from build123d import *

# Parameters (mm, degrees)
CYLINDER026_R             = 3
CYLINDER026_DEPTH         = 60
CYLINDER026_PITCH_ANGLE   = 90
CYLINDER025_R             = 3
CYLINDER025_DEPTH         = 100
CYLINDER025_ROLL_ANGLE    = 90
CYLINDER027_R             = 3
CYLINDER027_DEPTH         = 60
CYLINDER027_PITCH_ANGLE   = 90
FUSION011_PLACEMENT_ANGLE = 90
BOX026_W                  = 480
BOX026_H                  = 190
BOX026_DEPTH              = 15


with BuildPart() as cylinder032:
    # Cylinder026 → Cylinder026 (new body)
    with BuildSketch(Plane.XY):
        Circle(CYLINDER026_R)
    extrude(amount=CYLINDER026_DEPTH)


with BuildPart() as cylinder032_1:
    # Cylinder026 pitch: moved
    add(cylinder032.part.rotate(Axis((0, 0, 0), (0, 1, 0)), CYLINDER026_PITCH_ANGLE))


with BuildPart() as cylinder032_2:
    # Cylinder026 placement: moved
    add(cylinder032_1.part.moved(Location((-50, -3, 0))))


with BuildPart() as fusion010:
    # Cylinder025 → Cylinder025 (new body)
    with BuildSketch(Plane.XY):
        Circle(CYLINDER025_R)
    extrude(amount=CYLINDER025_DEPTH)


with BuildPart() as fusion010_1:
    # Cylinder025 roll: moved
    add(fusion010.part.rotate(Axis((0, 0, 0), (1, 0, 0)), CYLINDER025_ROLL_ANGLE))


with BuildPart() as fusion010_2:
    # Cylinder025 placement: moved
    add(fusion010_1.part.moved(Location((-50, 0, 0))))

    # Fusion010: union Cylinder032
    add(cylinder032_2.part)


with BuildPart() as handle_top:
    # Cylinder027 → Cylinder027 (new body)
    with BuildSketch(Plane.XY):
        Circle(CYLINDER027_R)
    extrude(amount=CYLINDER027_DEPTH)


with BuildPart() as handle_top_1:
    # Cylinder027 pitch: moved
    add(handle_top.part.rotate(Axis((0, 0, 0), (0, 1, 0)), CYLINDER027_PITCH_ANGLE))


with BuildPart() as handle_top_2:
    # Cylinder027 placement: moved
    add(handle_top_1.part.moved(Location((-50, -97, 0))))

    # Fusion011: union Fusion010
    add(fusion010_2.part)


with BuildPart() as handle_top_3:
    # Fusion011 placement: moved
    add(handle_top_2.part.moved(Location((195, 105, 299))).rotate(Axis((195, 105, 299), (0, 0, 1)), FUSION011_PLACEMENT_ANGLE))


with BuildPart() as solar_box_top_cover:
    # Box026 → Box026 (new body)
    with BuildSketch(Plane(origin=(10, 30, 285), x_dir=(1, 0, 0), z_dir=(0, 0, 1))):
        with Locations((240, 95)):
            Rectangle(BOX026_W, BOX026_H)
    extrude(amount=BOX026_DEPTH)

    # Fusion012: union Handle Top
    add(handle_top_3.part)


solid = solar_box_top_cover.part
CAD build for the part. Positions are in the model's coordinates, mm. Round coordinates to 2 decimals unless told otherwise and drop trailing zeros. Write each loop counter-clockwise with the first axis right and the second up, starting at its lowest first coordinate (ties: lowest second). Pieces come first, ordered by that corner, then holes.
(1) Drop flat-ended pins along their axis: P1, Ø5, axis at x = 219, y = 153, coming from the +Z side; P2, Ø0.6, axis at x = 197, z = 301.5, coming from the +Y side. Give the stop position or say it passes through.
(2) Slice it at A-A, the plane x = 217. Write the cut outline in (y, z), and give its area (3 significant figures).
(3) Slice it at D-D, the plane y = 182.5. Write the cut outline in (x, z), and give its area (3 significant figures).
(4) Slice it at C-C, the plane x = 322. Write the cut outline in (y, z).
(5) Slice it at B-B, the plane y = 74.5. Write the cut outline in (x, z), and give its area (3 significant figures).
(6) Probe line 1 along Z through (x, y) = (96, 204). List the from-to ranges inside material, lowest first.
From the geometry:
1. P1: stops at z = 300
1. P2: stops at y = 115
2. outline: (30, 285) - (220, 285) - (220, 300) - (57.83, 300) arc R3 ccw to (52.17, 300) - (30, 300) - close
2. area: 2,860 mm2
3. outline: (10, 285) - (490, 285) - (490, 300) - (10, 300) - close
3. area: 7,200 mm2
4. outline: (30, 285) - (220, 285) - (220, 300) - (30, 300) - close
5. outline: (10, 285) - (490, 285) - (490, 300) - (294.83, 300) arc R3 ccw to (289.17, 300) - (200.83, 300) arc R3 ccw to (195.17, 300) - (10, 300) - close
5. area: 7,220 mm2
6. line 1: z = 285 to 300
